Build history of the part. All positions in model axes, mm. Face numbers are marked on the shaded views. A direction names the side the tool comes from. Give positions to 0.01 mm unless a question says otherwise; leave off trailing zeros. Order: outer loops, then holes, each group sorted by start corner. A loop starts at its lowest first (then second) coordinate and runs counter-clockwise, first axis right, second up. Notation, with made-up numbers: M -14,21.25 L 29,21.25 A30 cw 29,50.25 Z; hole C 0.5,52.25 d7. An arc over 180 degrees is marked long. Answer as CSV lines item,"result".
from build123d import *

# Parameters (mm, degrees)
SKETCH1_W             = 15
SKETCH1_H             = 10
BOSS_EXTRUDE2_DEPTH   = 10
BOSS_EXTRUDE2_2_DEPTH = 10
BOSS_EXTRUDE3_DEPTH   = 10
FILLET1_R             = 0.2
FILLET2_R             = 1


with BuildPart() as part:
    # Sketch1 → Boss-Extrude2 (new body)
    with BuildSketch(Plane(origin=(0, 0, 0), x_dir=(1, 0, 0), z_dir=(0, 1, 0))):
        with Locations((0, 20)):
            Rectangle(SKETCH1_W, SKETCH1_H)
    extrude(amount=BOSS_EXTRUDE2_DEPTH)



with BuildPart() as body_2:
    # Sketch1 → Boss-Extrude2 2 (new body)
    with BuildSketch(Plane(origin=(0, 0, 0), x_dir=(1, 0, 0), z_dir=(0, 1, 0))):
        Rectangle(SKETCH1_W, SKETCH1_H)
    extrude(amount=BOSS_EXTRUDE2_2_DEPTH)


with BuildPart() as part_1:
    add(part.part)

    add(body_2.part)  # Boss-Extrude3 merges body 2
    # Sketch1<4> → Boss-Extrude3 (add)
    with BuildSketch(Plane(origin=(0, 0, 0), x_dir=(1, 0, 0), z_dir=(0, 1, 0))):
        Polygon((-12.5, 10), (0, 15), (-4.038873605, 15), (-16.538873605, 10), (-4.038873605, 5), (0, 5), align=None)
    boss_extrude3 = extrude(amount=BOSS_EXTRUDE3_DEPTH)

    # Mirror1: Boss-Extrude3 across plane
    add(boss_extrude3.mirror(Plane.ZY))

    # Fillet1
    fillet1_edges = [part_1.edges().sort_by_distance(p)[0] for p in [
        (-4.038873605, 5, -15),
        (-4.038873605, 5, -5),
        (0, 5, -5),
        (-12.5, 5, -10),
        (0, 5, -15),
        (4.038873605, 5, -15),
        (12.5, 5, -10),
        (4.038873605, 5, -5),
    ]]
    fillet(fillet1_edges, radius=FILLET1_R)

    # Fillet2
    fillet2_edges = [part_1.edges().sort_by_distance(p)[0] for p in [
        (-16.538873605, 5, -10),
        (16.538873605, 5, -10),
    ]]
    fillet(fillet2_edges, radius=FILLET2_R)


solid = part_1.part
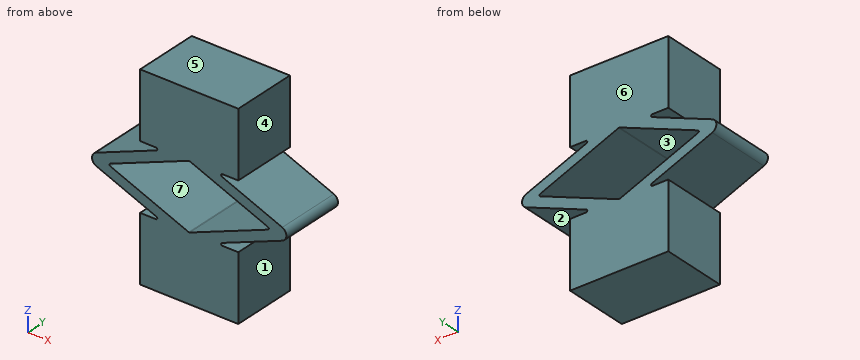
Item 1: Band-saw the part on B-B (y = 9). Give the cut face in (x, z).
Geometry says:
outline,"M -14.22,-10.93 L -5,-14.61 A0.2 cw -5.08,-15 L -7.5,-15 L -7.5,-25 L 7.5,-25 L 7.5,-15 L 5.08,-15 A0.2 cw 5,-14.61 L 14.22,-10.93 A1 ccw 14.22,-9.07 L 5,-5.39 A0.2 cw 5.08,-5 L 7.5,-5 L 7.5,5 L -7.5,5 L -7.5,-5 L -5.08,-5 A0.2 cw -5,-5.39 L -14.22,-9.07 A1 ccw Z; hole M -12.04,-10.19 L -0.07,-14.97 A0.2 ccw 0.07,-14.97 L 12.04,-10.19 A0.2 ccw 12.04,-9.81 L 0.07,-5.03 A0.2 ccw -0.07,-5.03 L -12.04,-9.81 A0.2 ccw Z"
Item 2: Pull direction Z, two halves, no side cores. Call the marked faces 5, 6 and 7: released by +Z, released by -Z, zero draft, split by the parting line, or undercut.
Geometry says:
face 5,"released by +Z"
face 6,"zero draft"
face 7,"undercut"
Item 3: Band-saw the part on D-D (z = -0.75). Give the cut face in (x, y).
Geometry says:
outline,"M -7.5,0 L 7.5,0 L 7.5,10 L -7.5,10 Z"
Item 4: Drop flat-ended pins along their axis: pin 1 (1.5 mm diameter, centred on x = 10.5, y = 8, fed in from +Z); pin 2 (8 mm diameter, centred on x = -4.5, z = -16.5, fed in from -Y); pin 3 (2 mm diameter, centred on y = 4, z = -8.5, fed in from -X); pin 4 (1 mm diameter, centred on x = -9.5, y = 7.5, fed in from -Z). Give the stop position or say it passes through.
Geometry says:
pin 1,"stops at z = -7.28"
pin 2,"stops at y = 0"
pin 3,"stops at x = -14.71"
pin 4,"stops at z = -13.02"
Item 5: Band-saw the part on C-C (z = -6.5). Give the cut face in (x, y).
Geometry says:
outline,"M -7.79,0 L -3.75,0 L -3.75,10 L -7.79,10 Z; M 3.75,0 L 7.79,0 L 7.79,10 L 3.75,10 Z"
Item 6: Probe line 1 along Z through (x, y) = (6.75, 3.75); line 2 along Z through (x, y) = (-5, 9); line 3 along X through (y, z) = (2.25, -23.25). List the from-to ranges inside material, lowest first. Write a range as from..to.
Geometry says:
line 1,"z = -25..-15, -13.92..-12.3, -7.7..-6.08, -5..5"
line 2,"z = -25..-14.98, -14.62..-13, -7..-5.38, -5.02..5"
line 3,"x = -7.5..7.5"
Item 7: 3-axis set-ups, long thin cutter, end or side, ignore diameter. For the marked faces 1, 2, 3 and 4: which of +Z, -Z, +X, -X, +Y, -Y reach the whole face in a straight line?
Geometry says:
face 1,"-Z, +X, +Y, -Y"
face 2,"+X, +Y, -Y"
face 3,"+Y, -Y"
face 4,"+Z, +X, +Y, -Y"
Item 8: Band-saw the part on A-A (x = -1). Give the cut face in (y, z).
Geometry says:
outline,"M 0,-25 L 10,-25 L 10,-14.6 L 0,-14.6 Z; M 0,-5.4 L 10,-5.4 L 10,5 L 0,5 Z"
